Check sheet for the drawn part. Datum: minimum x, y, z corner. Units: mm. A direction names the side the tool comes from. Round coordinates to 2 decimals unless told otherwise and drop trailing zeros. Loops run counter-clockwise (first coordinate to the right, second up) from the corner with the lowest first, then second, coordinate; pieces in that order, holes last.
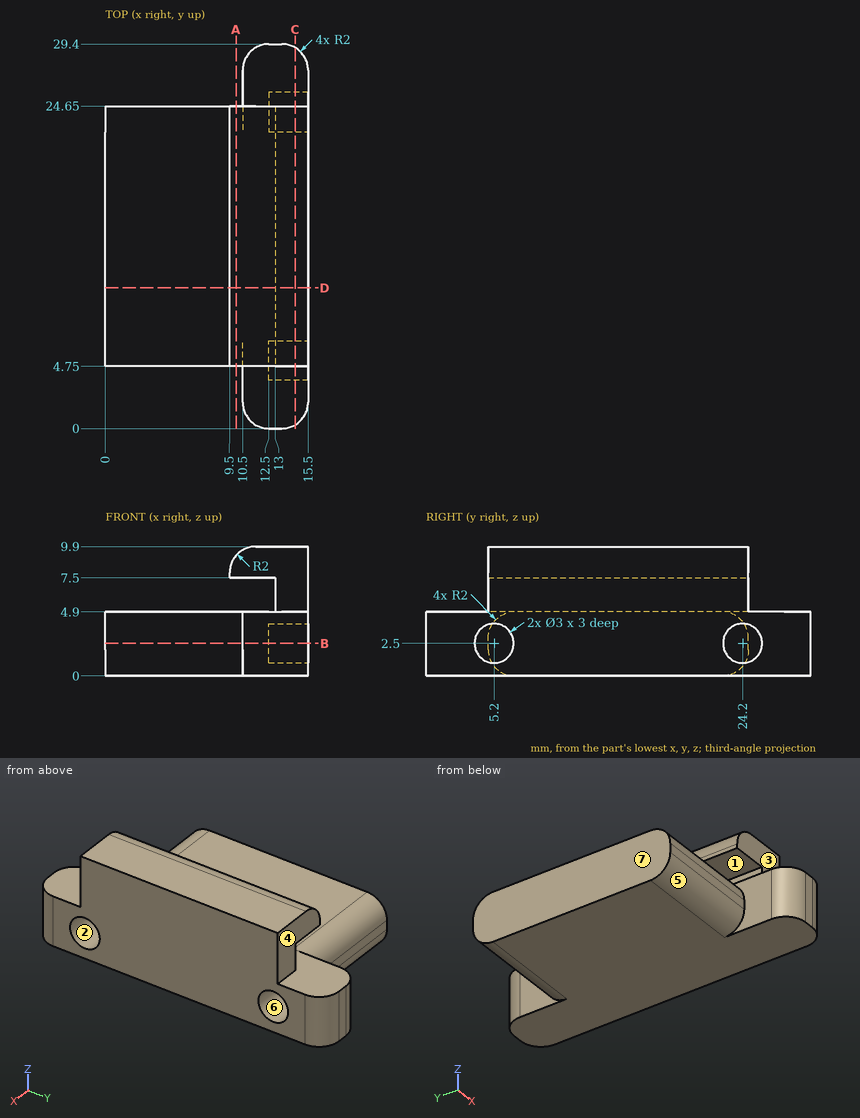
1) Sectioned sample at D-D, the plane y = 10.75. Record the cut outline in (x, z).
Report:
outline: (0, 0) - (15.5, 0) - (15.5, 9.9) - (11.5, 9.9) arc R2 ccw to (9.5, 7.9) - (9.5, 7.5) - (13, 7.5) - (13, 4.9) - (0, 4.9) - close
2) Sectioned sample at A-A, the plane x = 10. Record the cut outline in (y, z).
Report:
outline: (4.75, 2) arc R2 ccw to (6.75, 0) - (22.65, 0) arc R2 ccw to (24.65, 2) - (24.65, 2.9) arc R2 ccw to (22.65, 4.9) - (6.75, 4.9) arc R2 ccw to (4.75, 2.9) - close; (4.75, 7.5) - (24.65, 7.5) - (24.65, 9.22) - (4.75, 9.22) - close
3) Mould release check, pull along Z, two halves, no side actions. Record for the marked faces 5, 6 and 7: +Z half, -Z half, draft (parallel to the pull), parting line (faces both ways), or undercut.
Report:
face 5: -Z half
face 6: undercut
face 7: draft
4) Sectioned sample at B-B, the plane z = 2.5. Record the cut outline in (x, y), then the cut area to 3 significant figures.
Report:
outline: (0, 4.75) - (10.5, 4.75) - (10.5, 2) arc R2 ccw to (12.5, 0) - (13.5, 0) arc R2 ccw to (15.5, 2) - (15.5, 3.7) - (12.5, 3.7) - (12.5, 6.7) - (15.5, 6.7) - (15.5, 22.7) - (12.5, 22.7) - (12.5, 25.7) - (15.5, 25.7) - (15.5, 27.4) arc R2 ccw to (13.5, 29.4) - (12.5, 29.4) arc R2 ccw to (10.5, 27.4) - (10.5, 24.65) - (0, 24.65) - close
area: 335 mm2
5) Scan lines: line 1 along Z through (x, y) = (11.5, 18); line 2 along Z through (x, y) = (14.45, 24.2); line 3 along X through (y, z) = (5.25, 3.5). Record each from-to range of solid material in increasing order.
Report:
line 1: z = 0 to 4.9, 7.5 to 9.9
line 2: z = 0 to 1, 4 to 9.9
line 3: x = 0 to 12.5
6) Gauge pin test, flat ends, axial feed: pin 1 (1 mm diameter, centred on x = 3, z = 2.5, fed in from +Y); pin 2 (0.9 mm diameter, centred on y = 24, z = 3, fed in from +X); pin 3 (3 mm diameter, centred on y = 10, z = 6.5, fed in from -X). Record the tip position at first contact, or that the pin passes through.
Report:
pin 1: stops at y = 24.65
pin 2: stops at x = 12.5
pin 3: stops at x = 9.5
7) Access from +Z, -Z, +X, -X, +Y, -Y to the whole of each face (thin tool, end or side, straight path). Record for the marked faces 1, 2, 3 and 4.
Report:
face 1: -X, +Y, -Y
face 2: +X
face 3: +Z, +X, -X, -Y
face 4: +Z, +X, -X, +Y
8) Sectioned sample at C-C, the plane x = 14.5. Record the cut outline in (y, z).
Report:
outline: (0.27, 0) - (29.13, 0) - (29.13, 4.9) - (24.65, 4.9) - (24.65, 9.9) - (4.75, 9.9) - (4.75, 4.9) - (0.27, 4.9) - close; hole circle Ø3 at (5.2, 2.5); hole circle Ø3 at (24.2, 2.5)
